from build123d import *

# Parameters (mm, degrees)
SKETCH1_W             = 100
SKETCH1_H             = 30
SKETCH1_R             = 2.4892
SKETCH1_R_2           = 1.4986
SKETCH1_R_3           = 14
BOSS_EXTRUDE2_DEPTH   = 3.175
F_2_CLEARANCE_HOLE1_D = 2.4384
SKETCH5_R             = 4.7625
CUT_EXTRUDE1_DEPTH    = 105.45133137


with BuildPart() as part:
    # Sketch1 → Boss-Extrude2 (new body)
    with BuildSketch(Plane.XY):
        with Locations((50, 15)):
            Rectangle(SKETCH1_W, SKETCH1_H)
        with Locations((55, 15)):
            Circle(SKETCH1_R, mode=Mode.SUBTRACT)
        with Locations((37.166699296, 13)):
            Circle(SKETCH1_R_2, mode=Mode.SUBTRACT)
        with Locations((16, 15)):
            Circle(SKETCH1_R_3, mode=Mode.SUBTRACT)
    extrude(amount=BOSS_EXTRUDE2_DEPTH)

    # #2 Clearance Hole1 (through all)
    with Locations(Plane.XY.offset(3.175)):
        with Locations((97, 3), (97, 27), (3, 27), (3, 3), (34, 27), (34, 3)):
            Hole(F_2_CLEARANCE_HOLE1_D / 2)

    # Sketch5 → Cut-Extrude1 (cut, through all)
    with BuildSketch(Plane.XY.offset(3.175)):
        with Locations((85.9562, 15)):
            Circle(SKETCH5_R)
    extrude(amount=-CUT_EXTRUDE1_DEPTH, mode=Mode.SUBTRACT)


solid = part.part
Input: part model. Units: mm. Frame: model coordinates. Give positions to 0.01 mm unless a question says otherwise; leave off trailing zeros. Order: outer loops, then holes, each group sorted by start corner. A loop starts at its lowest first (then second) coordinate and runs counter-clockwise, first axis right, second up. Notation, with made-up numbers: (59.5, 18) - (111.5, 18) arc R16 cw to (111.5, 44) - close; hole circle Ø6 at (22.25, 6.5). An arc over 180 degrees is marked (long way). Answer as a JSON object with one key per item and string values. Group by question number.
Q1. Cut plane A-A, the plane x = 16. Output: boundary loops of the cut face in (y, z) (3 decimals), then the cut area to 3 significant figures.
Q2. Cut plane D-D, the plane y = 3. Output: boundary loops of the cut face in (x, z) (3 decimals), then the cut area to 3 significant figures.
Q3. First-contact query: pin 1 Ø3.5 at (x, y) = (37.17, 13) entering from +Z (3 decimals); pin 2 Ø2 at (x, y) = (34, 27) entering from -Z. Flat tips, straight axial feed; report the tip coordinate or a pass-through.
Q4. Cut plane C-C, the plane z = 1.15. Count the separate pieces of the cut face and the enclosed holes in it, then the cut area to 3 significant figures.
Q5. Cut plane B-B, the plane x = 34. Output: boundary loops of the cut face in (y, z) (3 decimals), then the cut area to 3 significant figures.
Q6. Mould query, pull axis X, two halves, no side actions, for faces 1 (the face through (2.437, 1.918, 1.565)), 2 (the face through (0, 15, 2)), 3 (the face through (60, 15, 3.175)). Classes: pulls with the +X half, pulls with the -X half, needs draft (parallel to the pull), parting line crosses it, or undercut.
Q7. Line query: probe 1 along Y at (x, z) = (34, 2.1); probe 2 along X at (y, z) = (15.25, 1.1); probe 3 along Y at (x, z) = (15.5, 2.8). Output: solid intervals per line, ascending.
Results:
{
 "1": {"outline": "(0, 0) - (1, 0) - (1, 3.175) - (0, 3.175) - close; (29, 0) - (30, 0) - (30, 3.175) - (29, 3.175) - close", "area": "6.35 mm^2"},
 "2": {"outline": "(0, 0) - (1.781, 0) - (1.781, 3.175) - (0, 3.175) - close; (4.219, 0) - (8.789, 0) - (8.789, 3.175) - (4.219, 3.175) - close; (23.211, 0) - (32.781, 0) - (32.781, 3.175) - (23.211, 3.175) - close; (35.219, 0) - (95.781, 0) - (95.781, 3.175) - (35.219, 3.175) - close; (98.219, 0) - (100, 0) - (100, 3.175) - (98.219, 3.175) - close", "area": "248 mm^2"},
 "3": {"pin 1": "z = 3.175", "pin 2": "through"},
 "4": {"separate pieces": "1", "enclosed holes": "10", "area": "2,260 mm^2"},
 "5": {"outline": "(0, 0) - (1.781, 0) - (1.781, 3.175) - (0, 3.175) - close; (4.219, 0) - (25.781, 0) - (25.781, 3.175) - (4.219, 3.175) - close; (28.219, 0) - (30, 0) - (30, 3.175) - (28.219, 3.175) - close", "area": "79.8 mm^2"},
 "6": {"face 1": "undercut", "face 2": "pulls with the -X half", "face 3": "needs draft"},
 "7": {"probe 1": "0 to 1.78, 4.22 to 25.78, 28.22 to 30", "probe 2": "0 to 2, 30 to 52.52, 57.48 to 81.2, 90.71 to 100", "probe 3": "0 to 1.01, 28.99 to 30"}
}
